```python
from build123d import *

# Parameters (mm, degrees)
BOX028_W          = 27
BOX028_H          = 14
BOX028_DEPTH      = 22
BOX009_W          = 80
BOX009_H          = 44
BOX009_DEPTH      = 8
BOX021_W          = 26
BOX021_H          = 26
BOX021_DEPTH      = 8
BOX020_W          = 26
BOX020_H          = 26
BOX020_DEPTH      = 8
CHAMFER017_SIZE   = 25
FILLET004003004_R = 1
FILLET004003005_R = 1.99
FILLET004003006_R = 3
CHAMFER033_SIZE   = 4
FILLET004003008_R = 3


with BuildPart() as cube028:
    # Box028 → Box028 (new body)
    with BuildSketch(Plane(origin=(59.5, -14, -7.5), x_dir=(1, 0, 0), z_dir=(0, 0, 1))):
        with Locations((13.5, 7)):
            Rectangle(BOX028_W, BOX028_H)
    extrude(amount=BOX028_DEPTH)


with BuildPart() as cube009:
    # Box009 → Box009 (new body)
    with BuildSketch(Plane(origin=(0, -14, 0), x_dir=(1, 0, 0), z_dir=(0, 0, 1))):
        with Locations((40, 22)):
            Rectangle(BOX009_W, BOX009_H)
    extrude(amount=BOX009_DEPTH)


with BuildPart() as cube021:
    # Box021 → Box021 (new body)
    with BuildSketch(Plane(origin=(-26, -39, 0), x_dir=(1, 0, 0), z_dir=(0, 0, 1))):
        with Locations((13, 13)):
            Rectangle(BOX021_W, BOX021_H)
    extrude(amount=BOX021_DEPTH)


with BuildPart() as fillet004003008:
    # Box020 → Box020 (new body)
    with BuildSketch(Plane(origin=(-1, -39, 0), x_dir=(1, 0, 0), z_dir=(0, 0, 1))):
        with Locations((13, 13)):
            Rectangle(BOX020_W, BOX020_H)
    extrude(amount=BOX020_DEPTH)

    # Chamfer017
    chamfer017_edges = [fillet004003008.edges().sort_by_distance(p)[0] for p in [
        (25, -39, 4),
    ]]
    chamfer(chamfer017_edges, length=CHAMFER017_SIZE)

    # Cut002008010: cut Cube021
    add(cube021.part, mode=Mode.SUBTRACT)

    # Fillet004003004
    fillet004003004_edges = [fillet004003008.edges().sort_by_distance(p)[0] for p in [
        (0, -39, 4),
    ]]
    fillet(fillet004003004_edges, radius=FILLET004003004_R)

    # Fusion006002011004053036004001003009006004: union Cube009
    add(cube009.part)

    # Fillet004003005
    fillet004003005_edges = [fillet004003008.edges().sort_by_distance(p)[0] for p in [
        (25, -14, 4),
    ]]
    fillet(fillet004003005_edges, radius=FILLET004003005_R)

    # Fillet004003006
    fillet004003006_edges = [fillet004003008.edges().sort_by_distance(p)[0] for p in [
        (80, -14, 4),
        (80, 30, 4),
        (0, 30, 4),
    ]]
    fillet(fillet004003006_edges, radius=FILLET004003006_R)

    # Cut002008023012003: cut Cube028
    add(cube028.part, mode=Mode.SUBTRACT)

    # Chamfer033
    chamfer033_edges = [fillet004003008.edges().sort_by_distance(p)[0] for p in [
        (59.5, -14, 4),
    ]]
    chamfer(chamfer033_edges, length=CHAMFER033_SIZE)

    # Fillet004003008
    fillet004003008_edges = [fillet004003008.edges().sort_by_distance(p)[0] for p in [
        (80, 0, 4),
    ]]
    fillet(fillet004003008_edges, radius=FILLET004003008_R)


solid = fillet004003008.part
```
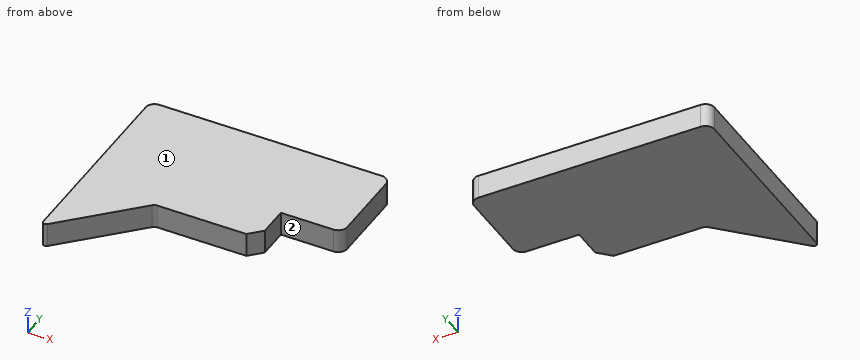
Geometry check sheet. Reference: the model listing, model coordinates, mm. Face numbers are marked on the shaded views. A direction names the side the tool comes from. Coordinates: 2 decimals unless noted, no trailing zeros. Order: outer loops, then holes, each group sorted by start corner. A loop starts at its lowest first (then second) coordinate and runs counter-clockwise, first axis right, second up. Notation, with made-up numbers: (22.5, -20.75) - (35.5, -20.75) arc R31 ccw to (35.5, 17.25) - close; hole circle Ø10 at (76, 45). An arc over 180 degrees is marked (long way). Answer as a JSON object with one key per item and string values. Group by question number.
Item 1: Sectioned sample at C-C, the plane x = 62.5. Record the cut outline in (y, z), and give its area (3 significant figures).
Item 2: Tool access check on the marked faces 1 and 2. Record the directions out of +Z, -Z, +X, -X, +Y, -Y that give a thin tool (end or side, any length) a straight path to the whole face; none if there is none.
Item 3: Sectioned sample at B-B, the plane y = -31.5. Record the cut outline in (x, z), and give its area (3 significant figures).
Item 4: Depth check by flat-ended pin: pin 1 Ø2.5 at (x, z) = (68, 5) entering from -Y; pin 2 Ø12 at (x, y) = (59.5, -14.5) entering from +Z; pin 3 Ø2.5 at (y, z) = (-4, 4.5) entering from +X. Enter the tip coordinate at first touch or a pass-through.
Item 5: Scan lines: probe 1 along Y at (x, z) = (43, 3.5); probe 2 along Y at (x, z) = (67, 3.75); probe 3 along X at (y, z) = (-22.5, 3.75). Record each from-to range of solid material in increasing order.
Item 6: Sectioned sample at A-A, the plane z = 5.5. Record the cut outline in (x, y).
Resolved:
{
 "1": {"outline": "(0, 0) - (30, 0) - (30, 8) - (0, 8) - close", "area": "240 mm^2"},
 "2": {"face 1": "+Z, +X, -X, +Y, -Y", "face 2": "+Z, -Z, +X, -Y"},
 "3": {"outline": "(0, 0) - (7.5, 0) - (7.5, 8) - (0, 8) - close", "area": "60.0 mm^2"},
 "4": {"pin 1": "y = 0", "pin 2": "z = 8", "pin 3": "x = 59.5"},
 "5": {"probe 1": "-14 to 30", "probe 2": "0 to 30", "probe 3": "0 to 16.5"},
 "6": {"outline": "(0, -36.59) arc R1 ccw to (1.71, -37.29) - (24.42, -14.58) arc R1.99 cw to (25.82, -14) - (55.5, -14) - (59.5, -10) - (59.5, 0) - (77, 0) arc R3 ccw to (80, 3) - (80, 27) arc R3 ccw to (77, 30) - (3, 30) arc R3 ccw to (0, 27) - close"}
}
